For this review, take the finished solid that the model builds, in its own axes (mm). Face numbers are marked on the shaded views. A direction names the side the tool comes from. Coordinates: 2 decimals unless noted, no trailing zeros. Order: outer loops, then holes, each group sorted by start corner. A loop starts at its lowest first (then second) coordinate and runs counter-clockwise, first axis right, second up.
from build123d import *

# Parameters (mm, degrees)
F0_W     = 29.845
F0_H     = 14.097
F0_W_2   = 2.5929864331
F0_H_2   = 1.524
F0_W_3   = 10.3421728662
F1_DEPTH = 1.524
F2_DEPTH = 15.875
F3_D     = 6.35
F3_DEPTH = 6.731
F3_TIP   = 1.9077324654
F4_R     = 3.048
F5_R     = 1.524


with BuildPart() as f1:
    # F0 (on Top) → F1 (new body)
    with BuildSketch(Plane.XY):
        Rectangle(F0_W, F0_H)
        Polygon((10.2975135669, 5.0165), (12.8905, 5.0165), (12.8905, 3.4925), (12.8905, -5.0165), (-12.8905, -5.0165), (-12.8905, 3.4925), (-12.8905, 5.0165), (-10.2975135669, 5.0165), (-5.1710864331, 5.0165), (5.1710864331, 5.0165), align=None, mode=Mode.SUBTRACT)
        Polygon((12.8905, -5.0165), (12.8905, 3.4925), (10.2975135669, 3.4925), (7.7343, 3.4925), (5.1710864331, 3.4925), (-5.1710864331, 3.4925), (-7.7343, 3.4925), (-10.2975135669, 3.4925), (-12.8905, 3.4925), (-12.8905, -5.0165), align=None)
        with Locations((11.5940067835, 4.2545)):
            Rectangle(F0_W_2, F0_H_2)
        Polygon((10.2975135669, 3.4925), (10.2975135669, 5.0165), (5.1710864331, 5.0165), (5.1710864331, 3.4925), (7.7343, 3.4925), align=None)
        with Locations((0, 4.2545)):
            Rectangle(F0_W_3, F0_H_2)
        Polygon((-5.1710864331, 3.4925), (-5.1710864331, 5.0165), (-10.2975135669, 5.0165), (-10.2975135669, 3.4925), (-7.7343, 3.4925), align=None)
        with Locations((-11.5940067835, 4.2545)):
            Rectangle(F0_W_2, F0_H_2)
    extrude(amount=F1_DEPTH)

    # F0 (on Top) → F2 (join)
    with BuildSketch(Plane.XY):
        Rectangle(F0_W, F0_H)
        Polygon((10.2975135669, 5.0165), (12.8905, 5.0165), (12.8905, 3.4925), (12.8905, -5.0165), (-12.8905, -5.0165), (-12.8905, 3.4925), (-12.8905, 5.0165), (-10.2975135669, 5.0165), (-5.1710864331, 5.0165), (5.1710864331, 5.0165), align=None, mode=Mode.SUBTRACT)
        Polygon((-5.1710864331, 3.4925), (-5.1710864331, 5.0165), (-10.2975135669, 5.0165), (-10.2975135669, 3.4925), (-7.7343, 3.4925), align=None)
        Polygon((10.2975135669, 3.4925), (10.2975135669, 5.0165), (5.1710864331, 5.0165), (5.1710864331, 3.4925), (7.7343, 3.4925), align=None)
    extrude(amount=F2_DEPTH)

    # F3
    with Locations(Plane(origin=(0, 0, 0), x_dir=(1, 0, 0), z_dir=(0, 0, -1))):
        with Locations((-7.7343, 0), (7.7343, 0)):
            Hole(F3_D / 2, depth=F3_DEPTH)
            with Locations((0, 0, -(F3_DEPTH + F3_TIP / 2))):  # 118° drill point
                Cone(0, F3_D / 2, F3_TIP, mode=Mode.SUBTRACT)

    # F4
    f4_edges = [f1.edges().sort_by_distance(p)[0] for p in [
        (-14.9225, 7.0485, 7.9375),
        (-14.9225, -7.0485, 7.9375),
        (14.9225, -7.0485, 7.9375),
        (14.9225, 7.0485, 7.9375),
    ]]
    fillet(f4_edges, radius=F4_R)

    # F5
    f5_edges = [f1.edges().sort_by_distance(p)[0] for p in [
        (0, -7.0485, 15.875),
        (0, 7.0485, 0),
    ]]
    fillet(f5_edges, radius=F5_R)


solid = f1.part
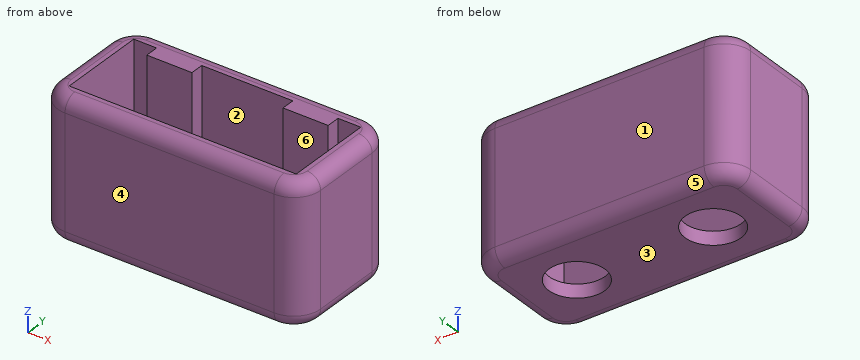
1. Take a section at B-B, the plane x = -5.75. Give the boundary of the cut face in (y, z) (1 decimal), plus the area to 3 significant figures.
Answer below:
outline: (-7, 1.5) arc R1.5 ccw to (-5.5, 0) - (-2.5, 0) - (-2.5, 1.5) - (-5, 1.5) - (-5, 15.9) - (-5.5, 15.9) arc R1.5 ccw to (-7, 14.4) - close; (2.5, 0) - (5.5, 0) arc R1.5 ccw to (7, 1.5) - (7, 14.4) arc R1.5 ccw to (5.5, 15.9) - (3.5, 15.9) - (3.5, 1.5) - (2.5, 1.5) - close
area: 92.1 mm2
2. Machinability: for the marked faces 1 and 2, which of the approach directions +Z, -Z, +X, -X, +Y, -Y give a long, thin tool a straight path to every point of the face, cutting with its end or side? Answer none if there is none.
Answer below:
face 1: +Z, -Z, +X, -X, +Y
face 2: +Z
3. Take a section at A-A, the plane y = 0. Give the boundary of the cut face in (x, z) (1 decimal), plus the area to 3 significant figures.
Answer below:
outline: (-14.9, 1.5) arc R1.5 ccw to (-13.4, 0) - (-10.9, 0) - (-10.9, 1.5) - (-12.9, 1.5) - (-12.9, 15.9) - (-13.4, 15.9) arc R1.5 ccw to (-14.9, 14.4) - close; (-4.6, 0) - (4.6, 0) - (4.6, 1.5) - (-4.6, 1.5) - close; (10.9, 0) - (13.4, 0) arc R1.5 ccw to (14.9, 1.5) - (14.9, 14.4) arc R1.5 ccw to (13.4, 15.9) - (12.9, 15.9) - (12.9, 1.5) - (10.9, 1.5) - close
area: 82.5 mm2
4. The part is to be moulded in two halves that separate along Y. For the marked faces 3, 4, 5 and 6, say which applies: +Y half, -Y half, draft (parallel to the pull), parting line (faces both ways), or undercut.
Answer below:
face 3: draft
face 4: -Y half
face 5: +Y half
face 6: undercut
5. Take a section at C-C, the plane z = 13.25. Give the boundary of the cut face in (x, y), plus the area to 3 significant figures.
Answer below:
outline: (-14.92, -4) arc R3.05 ccw to (-11.87, -7.05) - (11.87, -7.05) arc R3.05 ccw to (14.92, -4) - (14.92, 4) arc R3.05 ccw to (11.87, 7.05) - (-11.87, 7.05) arc R3.05 ccw to (-14.92, 4) - close; hole (-12.89, -5.02) - (12.89, -5.02) - (12.89, 5.02) - (10.3, 5.02) - (10.3, 3.49) - (5.17, 3.49) - (5.17, 5.02) - (-5.17, 5.02) - (-5.17, 3.49) - (-10.3, 3.49) - (-10.3, 5.02) - (-12.89, 5.02) - close
area: 170 mm2
6. To check wall thickness, follow L1, parallel to Y at x = 12, z = 7.75; L2, parallel to X at y = 4.5, z = 8; L3, parallel to Y at x = 5.5, z = 9. State the ranges of each line that lie inside material, in increasing order.
Answer below:
L1: y = -7.05 to -5.02, 5.02 to 7.05
L2: x = -14.88 to -12.89, -10.3 to -5.17, 5.17 to 10.3, 12.89 to 14.88
L3: y = -7.05 to -5.02, 3.49 to 7.05
7. Take a section at D-D, the plane x = 11.25. Give the boundary of the cut face in (y, z) (1 decimal).
Answer below:
outline: (-7, 1.5) arc R1.5 ccw to (-5.5, 0) - (5.5, 0) arc R1.5 ccw to (7, 1.5) - (7, 14.4) arc R1.5 ccw to (5.5, 15.9) - (5, 15.9) - (5, 1.5) - (-5, 1.5) - (-5, 15.9) - (-5.5, 15.9) arc R1.5 ccw to (-7, 14.4) - close
8. Clearance check with flat-ended pins moving along their axes: pin 1 Ø5 at (x, y) = (-7.73, 0) entering from +Z (1 decimal); pin 2 Ø5 at (x, y) = (1, 0) entering from +Z. State where each tip first meets the part, or that it passes through.
Answer below:
pin 1: passes through
pin 2: stops at z = 1.52
